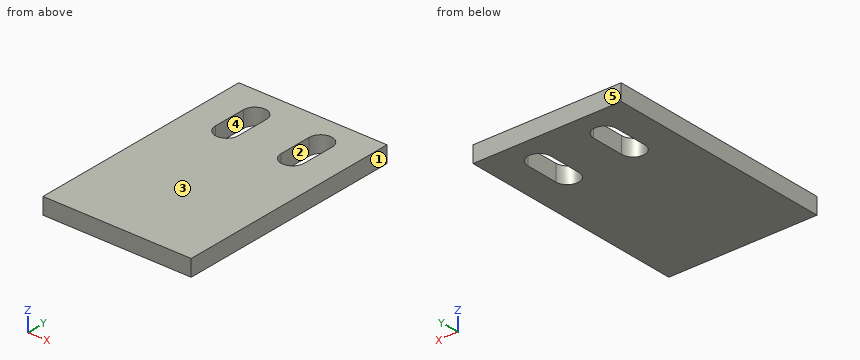
```python
from build123d import *

# Parameters (mm, degrees)
SKETCH_1_W             = 90
SKETCH_1_H             = 140
SM_BASE_FLANGE_1_DEPTH = 10


# Sheet-metal steps are written as plain solids
with BuildPart() as part:
    # Sketch 1 → Базовая кромка1 (new body)
    with BuildSketch(Plane.XY):
        with Locations((45, -70)):
            Rectangle(SKETCH_1_W, SKETCH_1_H)
        with BuildLine():
            Line((32, -18), (32, -38))
            ThreePointArc((32, -38), (25, -45), (18, -38))
            Line((18, -38), (18, -18))
            ThreePointArc((18, -18), (25, -11), (32, -18))
        make_face(mode=Mode.SUBTRACT)
        with BuildLine():
            Line((58, -18), (58, -38))
            ThreePointArc((58, -38), (65, -45), (72, -38))
            Line((72, -38), (72, -18))
            ThreePointArc((72, -18), (65, -11), (58, -18))
        make_face(mode=Mode.SUBTRACT)
    extrude(amount=-SM_BASE_FLANGE_1_DEPTH)


solid = part.part
```
Verification items for the finished model (mm, model axes). Face numbers are marked on the shaded views. A direction names the side the tool comes from. Round coordinates to 2 decimals unless told otherwise and drop trailing zeros. Order: outer loops, then holes, each group sorted by start corner. A loop starts at its lowest first (then second) coordinate and runs counter-clockwise, first axis right, second up. Notation, with made-up numbers: (42.5, 70) -> (101.5, 70) arc R31 cw to (101.5, 102) -> close; hole circle Ø10 at (88.25, -15). An arc over 180 degrees is marked (long way). Put each result on its own line as item: value. Start each with the question number.
(1) Section check B-B (y = -20). Enter the section's corners in (x, z).
(2) Draft check along X on the marked faces 1, 2 and 3. Enter one of: +X half, -X half, draft (parallel to the pull), parting line (faces both ways), or undercut.
(3) Tool access check on the marked faces 4 and 5. Record the directions out of +Z, -Z, +X, -X, +Y, -Y that give a thin tool (end or side, any length) a straight path to the whole face; none if there is none.
(4) Section check C-C (z = -1.5). Enter the section's corners in (x, y).
(5) Material ranges on line 1 along X through (y, z) = (-22, -3.5); line 2 along X through (y, z) = (-16, -9); line 3 along Y through (x, z) = (29, -4), recorded low to high.
(6) Section check A-A (x = 65). Enter the section's corners in (y, z), then the cut area to 3 significant figures.
(7) Section check D-D (x = 27). Enter the section's corners in (y, z), then the cut area to 3 significant figures.
Completed:
1. outline: (0, -10) -> (18, -10) -> (18, 0) -> (0, 0) -> close; (32, -10) -> (58, -10) -> (58, 0) -> (32, 0) -> close; (72, -10) -> (90, -10) -> (90, 0) -> (72, 0) -> close
2. face 1: +X half
2. face 2: undercut
2. face 3: draft
3. face 4: +Z, -Z
3. face 5: +Z, -Z, +X, -X, +Y
4. outline: (0, -140) -> (90, -140) -> (90, 0) -> (0, 0) -> close; hole (18, -38) arc R7 ccw to (32, -38) -> (32, -18) arc R7 ccw to (18, -18) -> close; hole (58, -38) arc R7 ccw to (72, -38) -> (72, -18) arc R7 ccw to (58, -18) -> close
5. line 1: x = 0 to 18, 32 to 58, 72 to 90
5. line 2: x = 0 to 18.29, 31.71 to 58.29, 71.71 to 90
5. line 3: y = -140 to -43.74, -12.26 to 0
6. outline: (-140, -10) -> (-45, -10) -> (-45, 0) -> (-140, 0) -> close; (-11, -10) -> (0, -10) -> (0, 0) -> (-11, 0) -> close
6. area: 1,060 mm2
7. outline: (-140, -10) -> (-44.71, -10) -> (-44.71, 0) -> (-140, 0) -> close; (-11.29, -10) -> (0, -10) -> (0, 0) -> (-11.29, 0) -> close
7. area: 1,070 mm2
